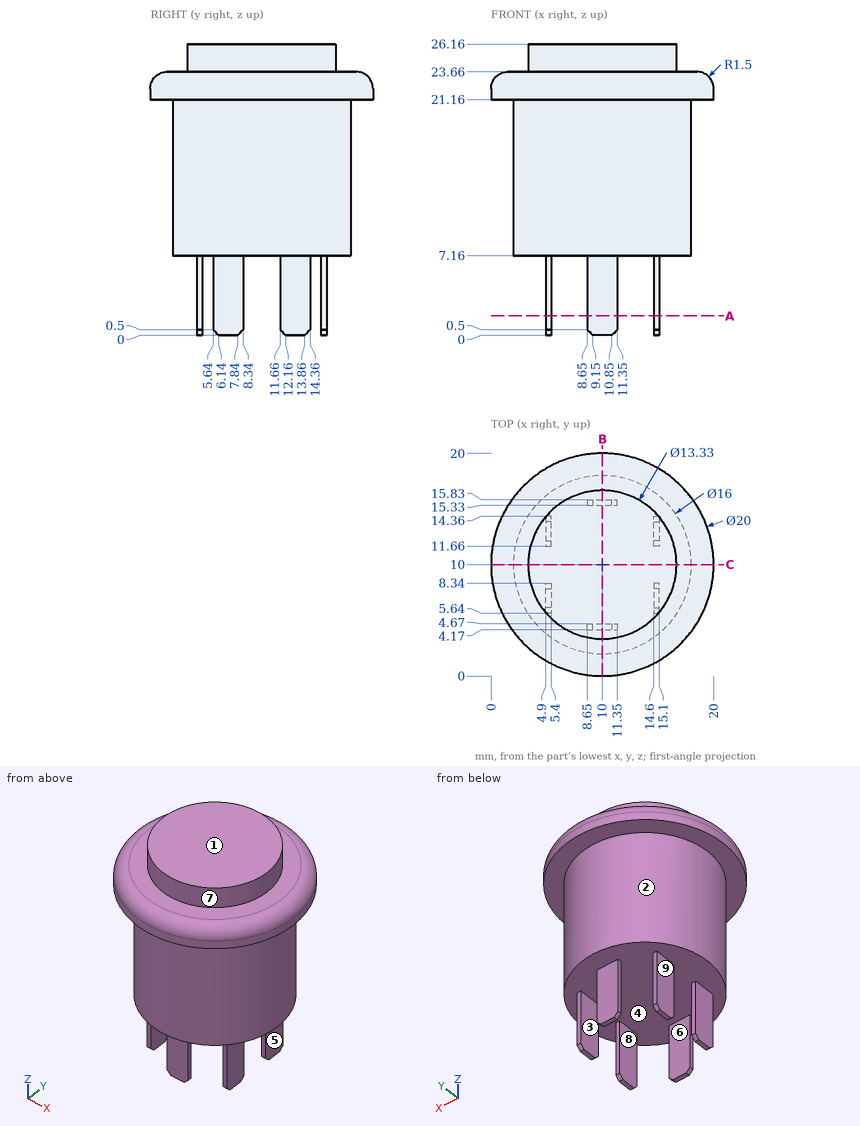
Source: three-view drawing plus pictorial views. Frame: mm from the lowest corner of the part. A direction names the side the tool comes from. Give positions to 0.01 mm unless a question says otherwise; leave off trailing zeros. Write each loop counter-clockwise with the first axis right and the second up, starting at its lowest first coordinate (ties: lowest second). Pieces come first, ordered by that corner, then holes. Notation, with made-up numbers: M -36.75,-19.75 L -16.75,-19.75 A22 cw -16.75,9.25 Z; hole C 6.25,0 d3. An arc over 180 degrees is marked long. Use one line per item in the form item = value.
1. Ray query, L1, parallel to X at y = 6.5, z = 5; L2, parallel to Z at x = 14, y = 2.75; L3, parallel to Y at x = 10, z = 4.25. Return the intervals inside material, ascending.
Outcome:
L1 = 4.9 to 5.4, 14.6 to 15.1
L2 = 21.16 to 23.66
L3 = 4.17 to 4.67, 15.33 to 15.83
2. Cut plane B-B on x = 10. Return loops of the section in (y, z) (3 decimals).
Outcome:
outline = M 0,21.16 L 2,21.16 L 2,7.16 L 4.17,7.16 L 4.17,0 L 4.67,0 L 4.67,7.16 L 15.33,7.16 L 15.33,0 L 15.83,0 L 15.83,7.16 L 18,7.16 L 18,21.16 L 20,21.16 L 20,22.16 A1.5 ccw 18.5,23.66 L 16.665,23.66 L 16.665,26.16 L 3.335,26.16 L 3.335,23.66 L 1.5,23.66 A1.5 ccw 0,22.16 Z
3. Mould query, pull axis X, two halves, no side actions, for the marked faces 1, 2, 3 and 4. Classes: released by +X, released by -X, zero draft, split by the parting line, or undercut.
Outcome:
face_1 = zero draft
face_2 = split by the parting line
face_3 = undercut
face_4 = undercut
4. Cut plane C-C on y = 10. Return loops of the section in (x, z) (3 decimals), and give its area (3 significant figures).
Outcome:
outline = M 0,21.16 L 2,21.16 L 2,7.16 L 18,7.16 L 18,21.16 L 20,21.16 L 20,22.16 A1.5 ccw 18.5,23.66 L 16.665,23.66 L 16.665,26.16 L 3.335,26.16 L 3.335,23.66 L 1.5,23.66 A1.5 ccw 0,22.16 Z
area = 306 mm²
5. Cut plane A-A on z = 1.75. Return loops of the section in (x, y), and give its area (3 significant figures).
Outcome:
outline = M 4.9,5.64 L 5.4,5.64 L 5.4,8.34 L 4.9,8.34 Z; M 4.9,11.66 L 5.4,11.66 L 5.4,14.36 L 4.9,14.36 Z; M 8.65,4.17 L 11.35,4.17 L 11.35,4.67 L 8.65,4.67 Z; M 8.65,15.33 L 11.35,15.33 L 11.35,15.83 L 8.65,15.83 Z; M 14.6,5.64 L 15.1,5.64 L 15.1,8.34 L 14.6,8.34 Z; M 14.6,11.66 L 15.1,11.66 L 15.1,14.36 L 14.6,14.36 Z
area = 8.10 mm²
6. Reachability of the marked faces 5, 6, 7, 8 and 9 from +Z, -Z, +X, -X, +Y, -Y: full face, straight path, thin tool, end or side. Return the list, or none.
Outcome:
face_5 = -Z, +X, +Y, -Y
face_6 = -Z, +X, -X
face_7 = +Z
face_8 = -Z, +Y, -Y
face_9 = -Z, -X, +Y, -Y
7. First-contact query: P1, Ø10, axis at y = 15.5, z = 21, coming from the +X side; P2, Ø1.5, axis at x = 2.5, z = 12, coming from the -Y side; P3, Ø0.8, axis at y = 7, z = 2, coming from the -X side. Flat tips, straight axial feed; report the tip coordinate or a pass-through.
Outcome:
P1 = 19.99
P2 = 5.71
P3 = 4.9
